The drawing under review shows one solid part. Ordinate dimensions are in mm from its lowest x, y, z. Give positions to 0.01 mm unless a question says otherwise; leave off trailing zeros. Loops run counter-clockwise (first coordinate to the right, second up) from the corner with the lowest first, then second, coordinate; pieces in that order, holes last. Notation, with made-up numbers: (0.5, -16.75) - (47.5, -16.75) arc R23 ccw to (47.5, -7.75) - close; hole circle Ø2 at (-16, -21). An arc over 180 degrees is marked (long way). Put each result on its own line as item: value. Start each with the question number.
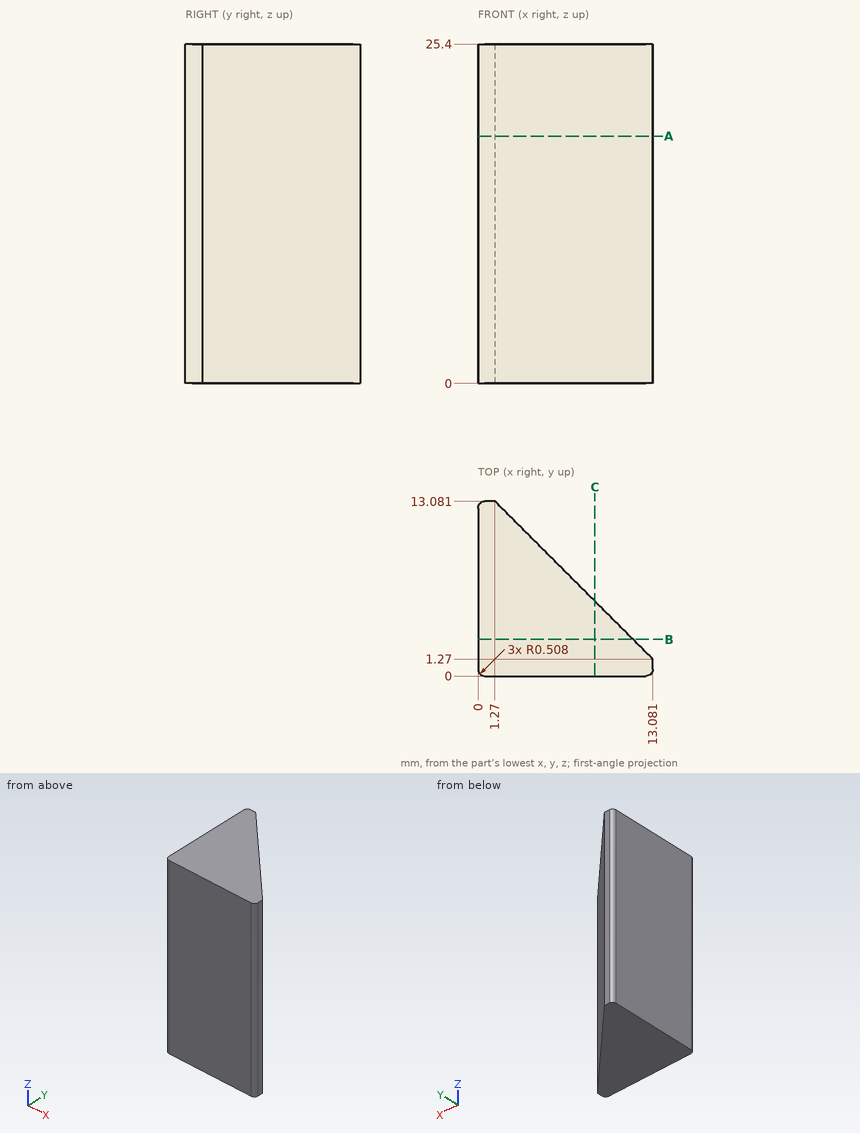
Item 1: Consider section C-C (x = 8.75). State the section outline as (y, z) points, plus the area to 3 significant figures.
Item 2: For P1, Ø6, axis at y = 4.5, z = 10.5, coming from the +X side; P2, Ø2, axis at x = 3.5, z = 14.5, coming from the +Y side; P3, Ø6, axis at y = 6, z = 19, coming from the +X side, all flat-tipped, find the tip position at first contact; note any pin that passes through.
Item 3: Consider section A-A (z = 18.5). State the section outline as (x, y) points.
Item 4: For L1, parallel to Y at x = 10.5, z = 19.5; L2, parallel to Y at x = 4.5, z = 8; L3, parallel to X at y = 10.75, z = 2.5, list the stretches that pass through material, from the lowest coordinate up. Write a range as from..to.
Item 5: Consider section B-B (y = 2.75). State the section outline as (x, z) points.
Geometry says:
1. outline: (0, 0) - (5.6, 0) - (5.6, 25.4) - (0, 25.4) - close
1. area: 142 mm2
2. P1: stops at x = 12.85
2. P2: stops at y = 11.85
2. P3: stops at x = 11.35
3. outline: (0, 0.51) arc R0.51 ccw to (0.51, 0) - (12.57, 0) arc R0.51 ccw to (13.08, 0.51) - (13.08, 1.27) - (1.27, 13.08) - (0.51, 13.08) arc R0.51 ccw to (0, 12.57) - close
4. L1: y = 0..3.85
4. L2: y = 0..9.85
4. L3: x = 0..3.6
5. outline: (0, 0) - (11.6, 0) - (11.6, 25.4) - (0, 25.4) - close
